Geometry: see drawing. Coordinates: mm, zero at the bounding-box minimum. Coordinates: 2 decimals unless noted, no trailing zeros. Write each loop counter-clockwise with the first axis right and the second up, starting at its lowest first coordinate (ties: lowest second). Pieces come first, ordered by that corner, then holes. Notation, with made-up numbers: (76, 9.25) - (103, 9.25) arc R23 ccw to (103, 20.25) - close; hole circle Ø5 at (30.5, 80.25). An arc over 180 degrees is marked (long way). Use CSV: the item, a comma, the result in double quotes.
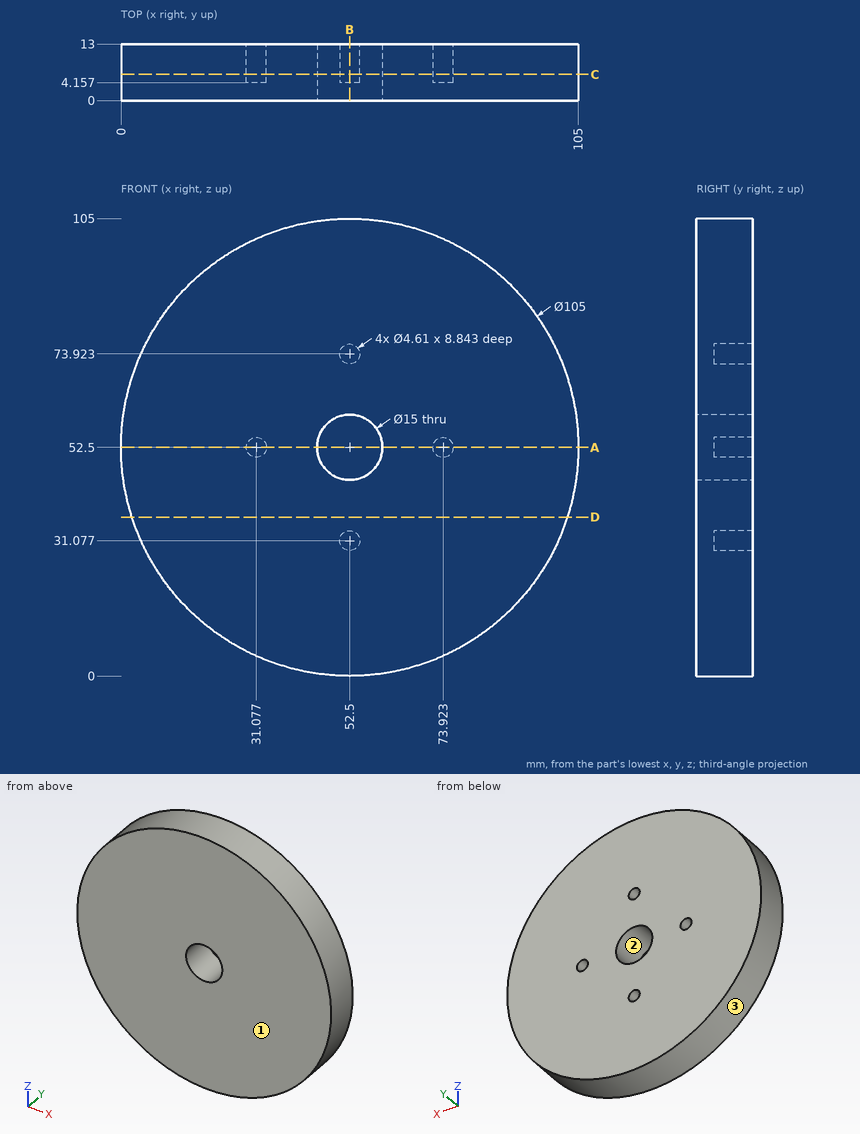
(1) Cut plane B-B on x = 52.5. Return loops of the section in (y, z), and give its area (3 significant figures).
Check values:
outline,"(0, 0) - (13, 0) - (13, 28.77) - (4.16, 28.77) - (4.16, 33.38) - (13, 33.38) - (13, 45) - (0, 45) - close; (0, 60) - (13, 60) - (13, 71.62) - (4.16, 71.62) - (4.16, 76.23) - (13, 76.23) - (13, 105) - (0, 105) - close"
area,"1,090 mm^2"
(2) Cut plane A-A on z = 52.5. Return loops of the section in (x, y), and give its area (3 significant figures).
Check values:
outline,"(0, 0) - (45, 0) - (45, 13) - (33.38, 13) - (33.38, 4.16) - (28.77, 4.16) - (28.77, 13) - (0, 13) - close; (60, 0) - (105, 0) - (105, 13) - (76.23, 13) - (76.23, 4.16) - (71.62, 4.16) - (71.62, 13) - (60, 13) - close"
area,"1,090 mm^2"
(3) Cut plane C-C on y = 6. Return loops of the section in (x, z) (1 decimal).
Check values:
outline,"circle Ø105 at (52.5, 52.5); hole circle Ø4.6 at (31.1, 52.5); hole circle Ø15 at (52.5, 52.5); hole circle Ø4.6 at (52.5, 31.1); hole circle Ø4.6 at (52.5, 73.9); hole circle Ø4.6 at (73.9, 52.5)"
(4) Pin query (flat end, axial travel): pin 1 Ø5 at (x, z) = (14, 68) entering from -Y; pin 2 Ø3 at (x, y) = (32.5, 10) entering from -Z; pin 3 Ø3 at (x, y) = (35, 2) entering from -Z; pin 4 Ø6 at (x, y) = (43.5, 10.5) entering from +Z. Return the tip coordinate at first contact, or that it passes through.
Check values:
pin 1,"y = 0"
pin 2,"z = 3.37"
pin 3,"z = 2.5"
pin 4,"z = 104.66"
(5) Cut plane D-D on z = 36.5. Return loops of the section in (x, y).
Check values:
outline,"(2.5, 0) - (102.5, 0) - (102.5, 13) - (2.5, 13) - close"
(6) Ray query, probe 1 along X at (y, z) = (9.75, 52.5); probe 2 along X at (y, z) = (4, 52.5); probe 3 along X at (y, z) = (10.5, 54.5) (1 decimal). Return the intervals inside material, ascending. Write a range as from..to.
Check values:
probe 1,"0..28.77, 33.38..45, 60..71.62, 76.23..105"
probe 2,"0..45, 60..105"
probe 3,"0..29.9, 32.2..45.3, 59.7..72.8, 75.1..105"
(7) Draft query along Z for the marked faces 1, 2 and 3. Return one class per face: pulls with the +Z half, pulls with the -Z half, needs draft (parallel to the pull), parting line crosses it, or undercut.
Check values:
face 1,"needs draft"
face 2,"undercut"
face 3,"parting line crosses it"
